The listing builds one solid part. Answer for the finished solid, in the listing's coordinates (mm). Coordinates: 2 decimals unless noted, no trailing zeros. Order: outer loops, then holes, each group sorted by start corner. A loop starts at its lowest first (then second) coordinate and runs counter-clockwise, first axis right, second up. Notation, with made-up numbers: M 54.5,57 L 109.5,57 A12 cw 109.5,74 Z; hole C 26.5,-30.75 d2. An arc over 180 degrees is marked long. One line per item, written item: value. Start each with the question number.
Q1. The part is cut by section C-C on y = 2.05. Give the vertices of the cut face in (x, z), then the cut area to 3 significant figures.
Q2. Straight lines are drawn through the part: line 1 along Y through (x, z) = (-25.5, -0.85); line 2 along X through (y, z) = (0.3, -0.25); line 3 along X through (y, z) = (-0.9, -0.8). For each, find the intervals that lie inside material, in ascending order. Write a range as [from, to].
Q3. The part is cut by section B-B on z = -0.4. Give the vertices of the cut face in (x, y), then the cut area to 3 significant figures.
Q4. The part is cut by section A-A on y = 0. Give the vertices of the cut face in (x, z), then the cut area to 4 significant figures.
Q5. The part is cut by section D-D on y = -1.7. Give the vertices of the cut face in (x, z), then the cut area to 3 significant figures.
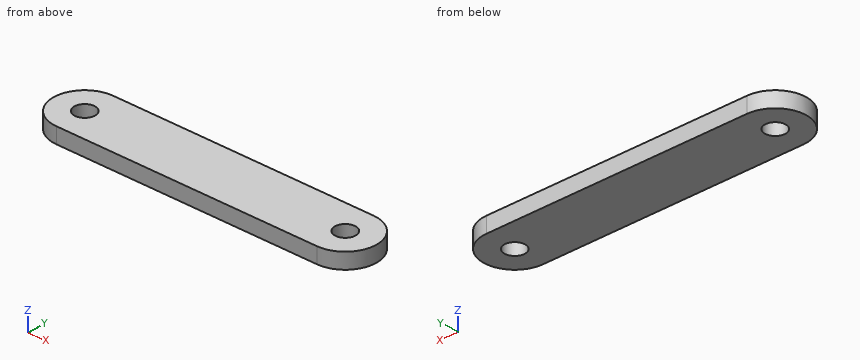
```python
from build123d import *

# Parameters (mm, degrees)
ESQUISSE1_R      = 1
EXTRUSION1_DEPTH = 1.5


with BuildPart() as part:
    # Esquisse1 → Extrusion1 (new body)
    with BuildSketch(Plane.XY):
        with BuildLine():
            Line((-25.5, 3), (0, 3))
            ThreePointArc((0, 3), (3, 0), (0, -3))
            Line((0, -3), (-25.5, -3))
            ThreePointArc((-25.5, -3), (-28.5, 0), (-25.5, 3))
        make_face()
        Circle(ESQUISSE1_R, mode=Mode.SUBTRACT)
        with Locations((-25.5, 0)):
            Circle(ESQUISSE1_R, mode=Mode.SUBTRACT)
    extrude(amount=-EXTRUSION1_DEPTH)


solid = part.part
```
Output:
1. outline: M -27.69,-1.5 L 2.19,-1.5 L 2.19,0 L -27.69,0 Z
1. area: 44.8 mm^2
2. line 1: y = [-3, -1], [1, 3]
2. line 2: x = [-28.48, -26.45], [-24.55, -0.95], [0.95, 2.98]
2. line 3: x = [-28.36, -25.94], [-25.06, -0.44], [0.44, 2.86]
3. outline: M -25.5,-3 L 0,-3 A3 ccw 0,3 L -25.5,3 A3 ccw Z; hole C -25.5,0 d2; hole C 0,0 d2
3. area: 175 mm^2
4. outline: M -28.5,-1.5 L -26.5,-1.5 L -26.5,0 L -28.5,0 Z; M -24.5,-1.5 L -1,-1.5 L -1,0 L -24.5,0 Z; M 1,-1.5 L 3,-1.5 L 3,0 L 1,0 Z
4. area: 41.25 mm^2
5. outline: M -27.97,-1.5 L 2.47,-1.5 L 2.47,0 L -27.97,0 Z
5. area: 45.7 mm^2
